Can you work these out from the model? Positions are in its coordinate system, mm. Face numbers are marked on the shaded views. A direction names the side the tool comes from. Give positions to 0.01 mm unless a question says otherwise; leave off trailing zeros. Loops run counter-clockwise (first coordinate to the right, second up) from the corner with the lowest first, then second, coordinate; pieces in that order, holes last. Notation, with made-up numbers: (18.5, 27) - (74.5, 27) arc R25 cw to (74.5, 43) - close; hole circle Ø11 at (-29.75, -31.75). An arc over 180 degrees is marked (long way). Answer in a Markdown table with one row per item.
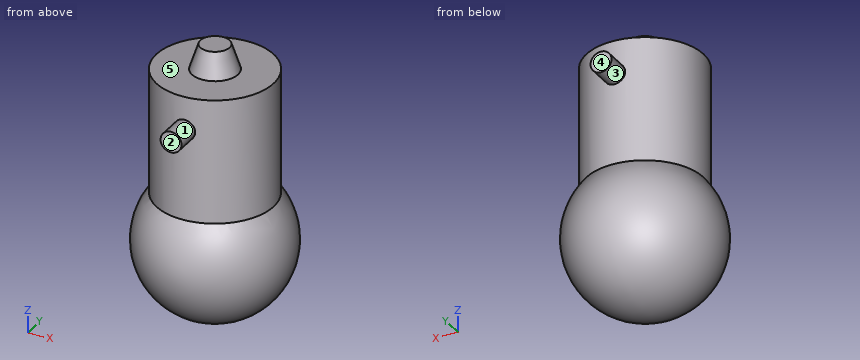
from build123d import *

# Parameters (mm, degrees)
ESQUISSE1_R        = 7
CORPS_DEPTH        = 15
ESQUISSE4_R        = 1.25
BAILLONETTES_DEPTH = 10


with BuildPart() as part:
    # Esquisse1 → Corps (new body)
    with BuildSketch(Plane.XY):
        with Locations(Location((0, 0, 0), (0, 0, 180))):  # turned: the seam where the file's is
            Circle(ESQUISSE1_R)
    extrude(amount=CORPS_DEPTH)

    # Esquisse3 → Verre (revolve)
    with BuildSketch(Plane(origin=(0, 0, 0), x_dir=(0, 0, -1), z_dir=(1, 0, 0))):
        with BuildLine():
            Line((5.5, -9), (5.5, 9))
            ThreePointArc((5.5, 9), (14.5, 0), (5.5, -9))
        make_face()
    revolve(axis=Axis((0, 11.000458592, -5.5), (0, -1, 0)))

    # Esquisse4 → Baillonettes (add, symmetric)
    with BuildSketch(Plane(origin=(0, 0, 0), x_dir=(1, 0, 0), z_dir=(0, 1, 0))):
        with Locations(Location((0, -11, 0), (0, 0, 90))):  # turned: the seam where the file's is
            Circle(ESQUISSE4_R)
    extrude(amount=BAILLONETTES_DEPTH, both=True)

    # Esquisse5 → Culot (revolve)
    with BuildSketch(Plane(origin=(0, 0, 0), x_dir=(0, 0, -1), z_dir=(1, 0, 0)), mode=Mode.PRIVATE) as culot_sk:
        Polygon((-18, 0), (-18, 1.75), (-15, 2.75), (-15, 0), align=None)
    revolve(culot_sk.sketch.rotate(Axis((0, 0, 9.557270233), (0, 0, 1)), 90), axis=Axis((0, 0, 9.557270233), (0, 0, 1)))  # turned: the seam where the file's is


solid = part.part
Q1. On a 3-axis mill with a long thin cutter (end or side, diameter ignored), from which of +Z, -Z, +X, -X, +Y, -Y can I reach the whole of each face in a straight line? I mean the marked faces 1, 2, 3, 4 and 5. Say none if no direction works.
Checked values:
| item | result |
|---|---|
| face 1 | -Y |
| face 2 | +Z, -Z, +X, -X, -Y |
| face 3 | +Y |
| face 4 | +Z, -Z, +X, -X, +Y |
| face 5 | +Z |
Q2. If I drill on line 1 (Y direction, x = -1, z = 10); line 2 (Z direction, x = -0.5, y = 6); line 3 (Z direction, x = 2.5, y = 1.5), over which ranges is the centre line in solid material (lowest first)? Write a range as [from, to].
Checked values:
| item | result |
|---|---|
| line 1 | y = [-6.93, 6.93] |
| line 2 | z = [-12.19, 15] |
| line 3 | z = [-14.01, 15] |
Q3. Imagine slicing it at B-B, the plane y = 0. Write out the boundary of the cut face in (x, z).
Checked values:
| item | result |
|---|---|
| outline | (-7, 0.16) arc R9 ccw (long way) to (7, 0.16) - (7, 15) - (2.75, 15) - (1.75, 18) - (-1.75, 18) - (-2.75, 15) - (-7, 15) - close |
Q4. Imagine slicing it at A-A, the plane z = 11. Write out the boundary of the cut face in (x, y), and give its area (3 significant figures).
Checked values:
| item | result |
|---|---|
| outline | (-1.25, -10) - (1.25, -10) - (1.25, -6.89) arc R7 ccw to (1.25, 6.89) - (1.25, 10) - (-1.25, 10) - (-1.25, 6.89) arc R7 ccw to (-1.25, -6.89) - close |
| area | 169 mm² |
Q5. Imagine slicing it at C-C, the plane y = 8. Write out the boundary of the cut face in (x, z).
Checked values:
| item | result |
|---|---|
| outline | circle Ø8.25 at (0, -5.5); circle Ø2.5 at (0, 11) |
Q6. For pin 1 (10 mm diameter, centred on y = -2, z = -9, fed in from +X); pin 2 (5 mm diameter, centred on y = 0, z = -9, fed in from -X); pin 3 (3 mm diameter, centred on y = -4.5, z = 14.5, fed in from -X); pin 4 (1 mm diameter, centred on x = 3.5, z = -3, fed in from -Y), each with a flat end and sliding along its axis, tell me the tip position at first contact or that it passes through.
Checked values:
| item | result |
|---|---|
| pin 1 | stops at x = 9 |
| pin 2 | stops at x = -8.94 |
| pin 3 | stops at x = -6.32 |
| pin 4 | stops at y = -8.16 |
Q7. Imagine slicing it at D-D, the plane x = 4. Write out the boundary of the cut face in (y, z), and give its area (3 significant figures).
Checked values:
| item | result |
|---|---|
| outline | (-5.74, 0.16) arc R8.06 ccw (long way) to (5.74, 0.16) - (5.74, 15) - (-5.74, 15) - close |
| area | 356 mm² |
